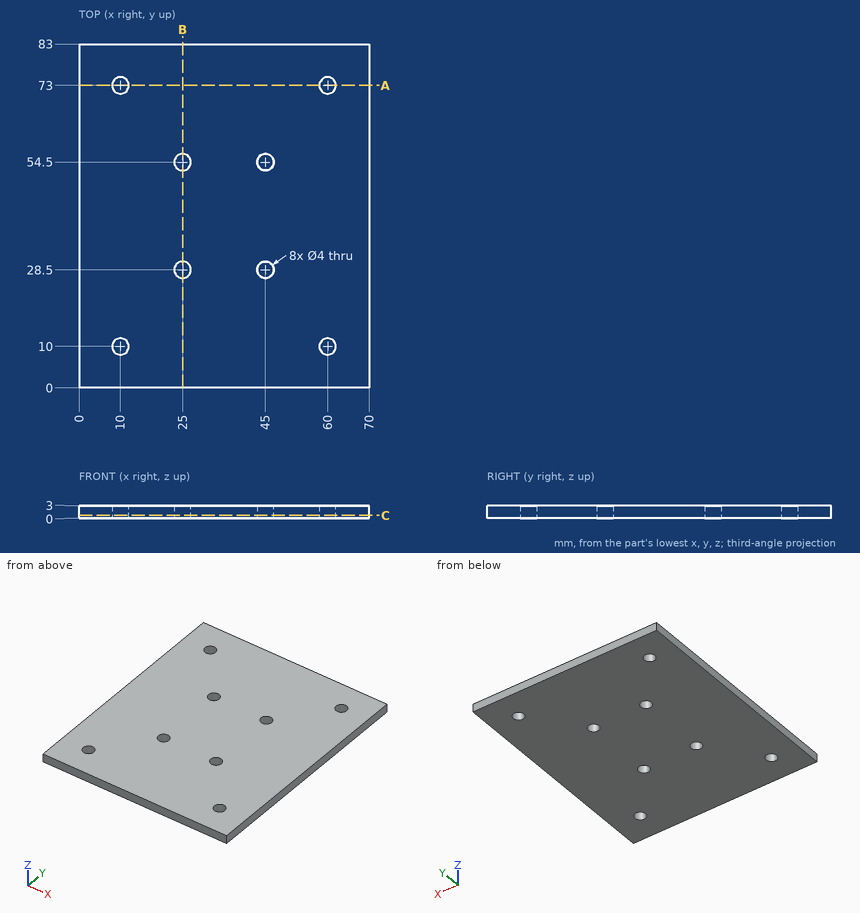
Geometry: see drawing. Coordinates: mm, zero at the bounding-box minimum. Give positions to 0.01 mm unless a question says otherwise; leave off trailing zeros. Order: outer loops, then holes, each group sorted by start corner. A loop starts at its lowest first (then second) coordinate and runs counter-clockwise, first axis right, second up. Notation, with made-up numbers: (-25.5, 25) - (22.5, 25) arc R9 ccw to (22.5, 31) - close; hole circle Ø6 at (88.25, 6.5). An arc over 180 degrees is marked (long way). Use CSV: the item, a comma, the result in double quotes.
1. Section query A-A (y = 73). Output: boundary loops of the cut face in (x, z), plus the area to 3 significant figures.
Answers below:
outline,"(0, 0) - (8, 0) - (8, 3) - (0, 3) - close; (12, 0) - (58, 0) - (58, 3) - (12, 3) - close; (62, 0) - (70, 0) - (70, 3) - (62, 3) - close"
area,"186 mm2"
2. Material intervals for line 1 along Y through (x, z) = (25, 1.85); line 2 along X through (y, z) = (55, 1.8); line 3 along X through (y, z) = (55.5, 0.65), sorted ascending. Write a range as from..to.
Answers below:
line 1,"0..26.5, 30.5..52.5, 56.5..83"
line 2,"0..23.06, 26.94..43.06, 46.94..70"
line 3,"0..23.27, 26.73..43.27, 46.73..70"
3. Section query C-C (z = 0.7). Give the number of separate pieces and of enclosed holes in the cut face, plus the area to 3 significant figures.
Answers below:
separate pieces,"1"
enclosed holes,"8"
area,"5,710 mm2"
4. Contact query for a flat-ended pin moving along its axis: pin 1 (10 mm diameter, centred on x = 30.5, y = 54.5, fed in from -Z). Output: stop coordinate, or through.
Answers below:
pin 1,"z = 0"
5. Section query B-B (x = 25). Output: boundary loops of the cut face in (y, z), plus the area to 3 significant figures.
Answers below:
outline,"(0, 0) - (26.5, 0) - (26.5, 3) - (0, 3) - close; (30.5, 0) - (52.5, 0) - (52.5, 3) - (30.5, 3) - close; (56.5, 0) - (83, 0) - (83, 3) - (56.5, 3) - close"
area,"225 mm2"
